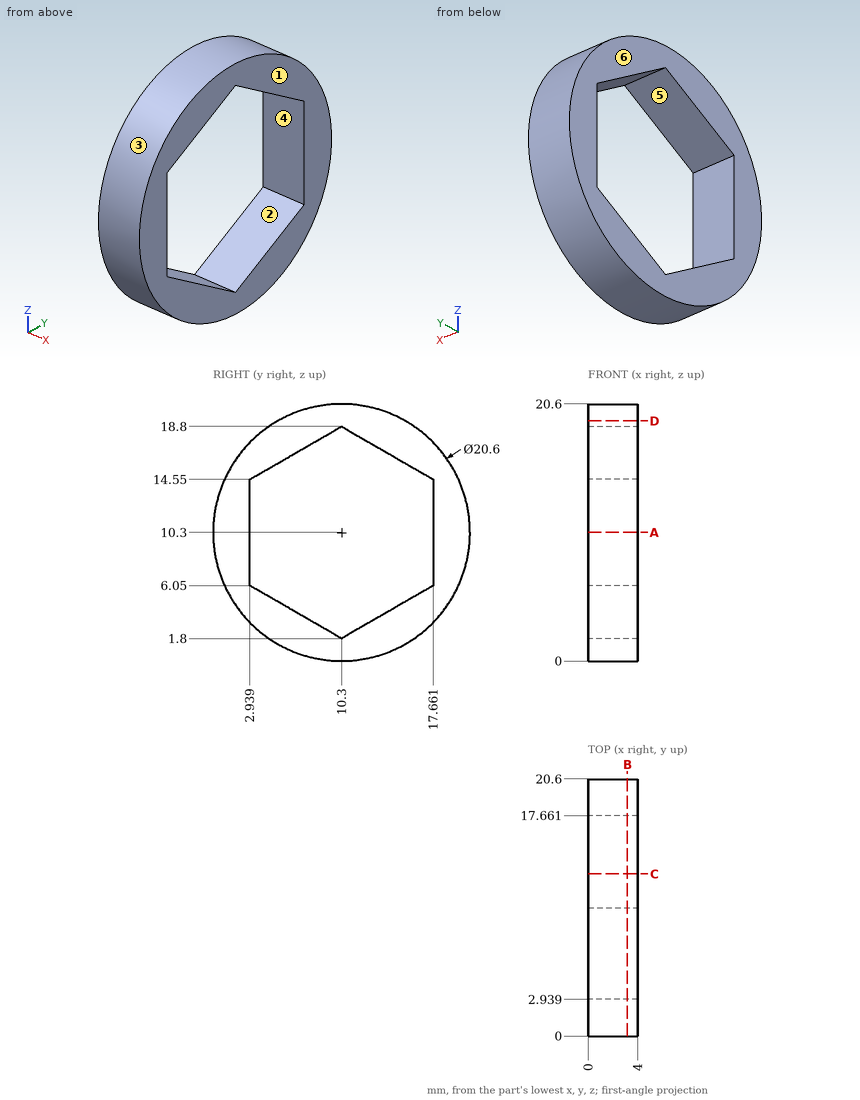
The drawing under review shows one solid part. Ordinate dimensions are in mm from its lowest x, y, z. A direction names the side the tool comes from. Coordinates: 2 decimals unless noted, no trailing zeros. Order: outer loops, then holes, each group sorted by start corner. A loop starts at its lowest first (then second) coordinate and runs counter-clockwise, first axis right, second up. Notation, with made-up numbers: (-34.5, 88) -> (-30.5, 88) arc R17 cw to (-30.5, 92) -> close; hole circle Ø4 at (57.5, -37). An arc over 180 degrees is marked (long way). Answer in a Markdown table with one row per item.
(1) Machinability: for the marked faces 5 and 6, which of the approach directions +Z, -Z, +X, -X, +Y, -Y give a long, thin tool a straight path to every point of the face, cutting with its end or side? Answer none if there is none.
Answers:
| item | result |
|---|---|
| face 5 | +X, -X |
| face 6 | +Z, -Z, -X, +Y, -Y |
(2) Consider section A-A (z = 10.3). Write out the cut boundary in (x, y), plus the area to 3 significant figures.
Answers:
| item | result |
|---|---|
| outline | (0, 0) -> (4, 0) -> (4, 2.94) -> (0, 2.94) -> close; (0, 17.66) -> (4, 17.66) -> (4, 20.6) -> (0, 20.6) -> close |
| area | 23.5 mm² |
(3) Wall thickness on line 1 along Y through (x, z) = (1.4, 10); line 2 along Y through (x, z) = (1.65, 5); line 3 along Z through (x, y) = (1.35, 17): over which ranges is each line inside the solid? List them lowest first.
Answers:
| item | result |
|---|---|
| line 1 | 0 to 2.94, 17.66 to 20.6 |
| line 2 | 1.47 to 4.76, 15.84 to 19.13 |
| line 3 | 2.48 to 5.67, 14.93 to 18.12 |
(4) The part is to be moulded in two halves that separate along Y. For the marked faces 1, 2, 3 and 4, say which applies: +Y half, -Y half, draft (parallel to the pull), parting line (faces both ways), or undercut.
Answers:
| item | result |
|---|---|
| face 1 | draft |
| face 2 | undercut |
| face 3 | parting line |
| face 4 | undercut |
(5) Consider section B-B (x = 3.15). Write out the cut boundary in (y, z), plus the area to 3 significant figures.
Answers:
| item | result |
|---|---|
| outline | circle Ø20.6 at (10.3, 10.3); hole (2.94, 6.05) -> (10.3, 1.8) -> (17.66, 6.05) -> (17.66, 14.55) -> (10.3, 18.8) -> (2.94, 14.55) -> close |
| area | 146 mm² |
(6) Consider section D-D (z = 19.25). Write out the cut boundary in (x, y).
Answers:
| item | result |
|---|---|
| outline | (0, 5.2) -> (4, 5.2) -> (4, 15.4) -> (0, 15.4) -> close |
(7) Insertion check: pin 1 (2 mm diameter, centred on x = 0.5, y = 18.5, fed in from -Z) (1 decimal); pin 2 (2 mm diameter, centred on x = 1.5, z = 8.5, fed in from +Y); pin 3 (1.2 mm diameter, centred on x = 2.5, z = 11.5, fed in from -Y). Each pin has a flat end and moves straight along its axis. Give the tip position at first contact, or say it passes through.
Answers:
| item | result |
|---|---|
| pin 1 | z = 2.9 |
| pin 2 | y = 20.57 |
| pin 3 | y = 0.02 |
(8) Consider section C-C (y = 13). Write out the cut boundary in (x, z), plus the area to 3 significant figures.
Answers:
| item | result |
|---|---|
| outline | (0, 0.36) -> (4, 0.36) -> (4, 3.36) -> (0, 3.36) -> close; (0, 17.24) -> (4, 17.24) -> (4, 20.24) -> (0, 20.24) -> close |
| area | 24.0 mm² |
